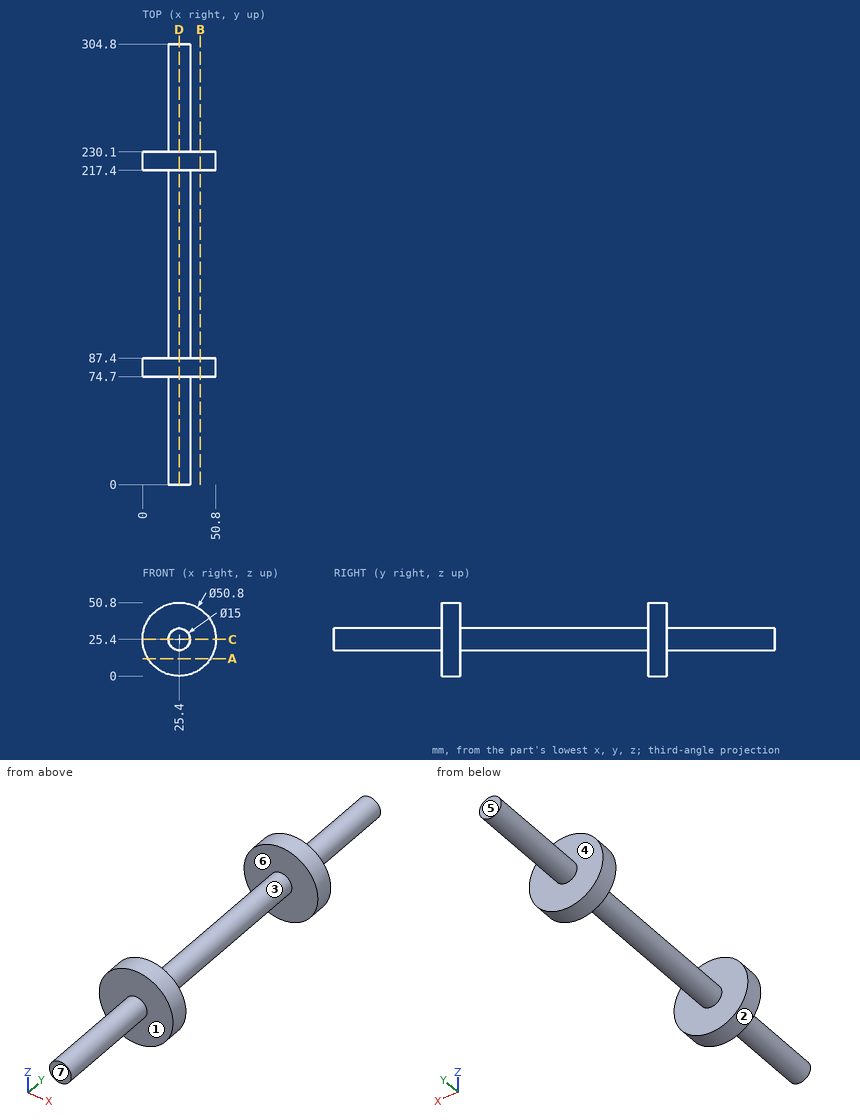
Study the drawing (mm; zero at the part's minimum x, y, z) and answer. A direction names the side the tool comes from. Round coordinates to 2 decimals unless told otherwise and drop trailing zeros. Loops run counter-clockwise (first coordinate to the right, second up) from the corner with the lowest first, then second, coordinate; pieces in that order, holes last.
Q1. Section B-B, the plane x = 40 is taken. Determine the outline of the cut face in (y, z), then the cut area to 3 significant figures.
Q2. For a pull along Y with two mould halves and no side action, classify the marked faces 5, 6 and 7 as released by +Y, released by -Y, zero draft, split by the parting line, or undercut.
Q3. Which of the six approach directions +Z, -Z, +X, -X, +Y, -Y give full straight-line access (tool end or side, diameter ignored) to the marked faces 1, 2, 3 and 4?
Q4. Section C-C, the plane z = 25.4 is taken. Determine the outline of the cut face in (x, y).
Q5. Find the intervals of material crossed by line 1 (Y direction, x = 35, z = 9); line 2 (X direction, y = 30, z = 27.5); line 3 (X direction, y = 224, z = 11.5), in increasing order.
Q6. Section A-A, the plane z = 12 is taken. Determine the outline of the cut face in (x, y).
Q7. Given pin 1 Ø12 at (x, z) = (14.5, 39) entering from -Y; pin 2 Ø6 at (x, z) = (36, 21) entering from +Y; pin 3 Ø2 at (x, z) = (21, 22.5) entering from -Y; pin 4 Ø1.5 at (y, z) = (128.5, 24.5) entering from -X, each flat-ended and moving along its own axis, determine where each tip first touches the part or whether it passes through.
Q8. Section D-D, the plane x = 25.4 is taken. Determine the outline of the cut face in (y, z).
Completed:
1. outline: (74.7, 4.62) - (87.4, 4.62) - (87.4, 46.18) - (74.7, 46.18) - close; (217.4, 4.62) - (230.1, 4.62) - (230.1, 46.18) - (217.4, 46.18) - close
1. area: 1,060 mm2
2. face 5: released by +Y
2. face 6: undercut
2. face 7: released by -Y
3. face 1: -Y
3. face 2: +Y, -Y
3. face 3: none
3. face 4: +Y
4. outline: (0, 74.7) - (17.9, 74.7) - (17.9, 0) - (32.9, 0) - (32.9, 74.7) - (50.8, 74.7) - (50.8, 87.4) - (32.9, 87.4) - (32.9, 217.4) - (50.8, 217.4) - (50.8, 230.1) - (32.9, 230.1) - (32.9, 304.8) - (17.9, 304.8) - (17.9, 230.1) - (0, 230.1) - (0, 217.4) - (17.9, 217.4) - (17.9, 87.4) - (0, 87.4) - close
5. line 1: y = 74.7 to 87.4, 217.4 to 230.1
5. line 2: x = 18.2 to 32.6
5. line 3: x = 4.14 to 46.66
6. outline: (3.82, 74.7) - (46.98, 74.7) - (46.98, 87.4) - (3.82, 87.4) - close; (3.82, 217.4) - (46.98, 217.4) - (46.98, 230.1) - (3.82, 230.1) - close
7. pin 1: stops at y = 74.7
7. pin 2: stops at y = 230.1
7. pin 3: stops at y = 0
7. pin 4: stops at x = 17.9
8. outline: (0, 17.9) - (74.7, 17.9) - (74.7, 0) - (87.4, 0) - (87.4, 17.9) - (217.4, 17.9) - (217.4, 0) - (230.1, 0) - (230.1, 17.9) - (304.8, 17.9) - (304.8, 32.9) - (230.1, 32.9) - (230.1, 50.8) - (217.4, 50.8) - (217.4, 32.9) - (87.4, 32.9) - (87.4, 50.8) - (74.7, 50.8) - (74.7, 32.9) - (0, 32.9) - close
